```python
from build123d import *

# Parameters (mm, degrees)
BOSS_EXTRUDE1_DEPTH = 19.05
BOSS_EXTRUDE2_DEPTH = 3.175
SKETCH3_R           = 3.175
CUT_EXTRUDE1_DEPTH  = 189.387669682
SKETCH4_W           = 151.529186582
SKETCH4_H           = 154.937341475
CUT_EXTRUDE2_DEPTH  = 146.05


with BuildPart() as part:
    # Sketch1 → Boss-Extrude1 (new body)
    with BuildSketch(Plane.XY):
        Polygon((0, 0), (0, -26.595904174), (100.162396017, -140.692505), (127, -140.692505), (127, -137.517505), (101.6, -137.517505), (3.175, -25.4), (3.175, 0), align=None)
    boss_extrude1 = extrude(amount=BOSS_EXTRUDE1_DEPTH)

    # Sketch2 → Boss-Extrude2 (add)
    with BuildSketch(Plane(origin=(0, 0, 0), x_dir=(-1, 0, 0), z_dir=(0, 0, -1))):
        Polygon((-19.05, 0), (-3.175, 0), (-3.175, -25.4), (-101.6, -137.517505), (-127, -137.517505), (-127, -121.642505), (-108.788019913, -121.642505), (-19.05, -19.42047913), align=None)
    boss_extrude2 = extrude(amount=-BOSS_EXTRUDE2_DEPTH)

    # Sketch3 → Cut-Extrude1 (cut, through all)
    with BuildSketch(Plane(origin=(3.175, 0, 0), x_dir=(0, 0, -1), z_dir=(1, 0, 0))):
        with Locations(Location((-11.1125, -7.690689216, 0), (0, 0, 90))):
            Circle(SKETCH3_R)
    cut_extrude1 = extrude(amount=-CUT_EXTRUDE1_DEPTH, mode=Mode.SUBTRACT)

    # Mirror1: Boss-Extrude1, Boss-Extrude2, Cut-Extrude1 across plane
    add(boss_extrude1.mirror(Plane(origin=(0, 0, 19.05), x_dir=(0, 0, 1), z_dir=(1, 0, 0))))
    add(boss_extrude2.mirror(Plane(origin=(0, 0, 19.05), x_dir=(0, 0, 1), z_dir=(1, 0, 0))))
    add(cut_extrude1.mirror(Plane(origin=(0, 0, 19.05), x_dir=(0, 0, 1), z_dir=(1, 0, 0))), mode=Mode.SUBTRACT)

    # Sketch4 → Cut-Extrude2 (cut)
    with BuildSketch(Plane.XY.offset(19.05)):
        with Locations((75.764593291, -77.468670738)):
            Rectangle(SKETCH4_W, SKETCH4_H)
    extrude(amount=-CUT_EXTRUDE2_DEPTH, mode=Mode.SUBTRACT)


solid = part.part
```
The model under review builds one solid part; all positions refer to its coordinate system, in mm. A direction names the side the tool comes from. Coordinates: 2 decimals unless noted, no trailing zeros. Write each loop counter-clockwise with the first axis right and the second up, starting at its lowest first coordinate (ties: lowest second). Pieces come first, ordered by that corner, then holes. Notation, with made-up numbers: (72, 57.5) - (89, 57.5) arc R16 ccw to (89, 69.5) - close; hole circle Ø1 at (-1, -15). An arc over 180 degrees is marked (long way). Answer in a Markdown table with one row per item. Add a question column.
Q1. Consider section A-A on z = 16.5. Give the boundary of the cut face in (x, y) (1 decimal).
Q2. To check wall thickness, follow line 1 along Z through (x, y) = (-102, -118) (3 decimals); line 2 along X through (y, z) = (-13, 4) (3 decimals); line 3 along Y through (x, z) = (-113, 13.5). State the ranges of each line that lie inside material, in increasing order. Write a range as from..to.
Q3. Draft analysis for pull direction Z (two halves, no side actions). For faces 4 (the face through (-56, -74, 3.175)), 5 (the face through (-7, 0, 2)), 6 (the face through (-1.61, -10.21, 9.18)), state which applies: +Z half, -Z half, draft (parallel to the pull), parting line (faces both ways), or undercut.
Q4. Clearance check with flat-ended pins moving along their axes: pin 1 (3.5 mm diameter, centred on x = -122, z = 1.5, fed in from +Y); pin 2 (2 mm diameter, centred on x = -96, z = 13.5, fed in from -Y); pin 3 (5 mm diameter, centred on x = -109, z = 11, fed in from +Y). State where each tip first meets the part, or that it passes through.
Q5. Consider section D-D on y = -111. Give the boundary of the cut face in (x, z) (3 decimals).
Q6. Consider section B-B on z = 9.5. Give the boundary of the cut face in (x, y) (1 decimal), then the cut area to 3 significant figures.
Q7. For faces 1 (the face through (-114, -137.518, 11)), 2 (the face through (-127, -138, 5)), 3 (the face through (-19.05, -10, 2)), list the 3-axis set-ups (+Z, -Z, +X, -X, +Y, -Y) from which the entire face can be reached by the end or side of a thin tool; tool diameter is ignored.
Answers below:
| question | item | result |
|---|---|---|
| 1 | outline | (-127, -140.7) - (-100.2, -140.7) - (0, -26.6) - (0, 0) - (-3.2, 0) - (-3.2, -25.4) - (-101.6, -137.5) - (-127, -137.5) - close |
| 2 | line 1 | 0..3.175 |
| 2 | line 2 | -3.175..0 |
| 2 | line 3 | -140.69..-137.52 |
| 3 | face 4 | +Z half |
| 3 | face 5 | draft |
| 3 | face 6 | undercut |
| 4 | pin 1 | y = -121.64 |
| 4 | pin 2 | y = -137.09 |
| 4 | pin 3 | y = -137.52 |
| 5 | outline | (-99.445, 0) - (-74.096, 0) - (-74.096, 19.05) - (-78.321, 19.05) - (-78.321, 3.175) - (-99.445, 3.175) - close |
| 6 | outline | (-127, -140.7) - (-100.2, -140.7) - (0, -26.6) - (0, -10.4) - (-3.2, -10.4) - (-3.2, -25.4) - (-101.6, -137.5) - (-127, -137.5) - close; (-3.2, -5) - (0, -5) - (0, 0) - (-3.2, 0) - close |
| 6 | area | 626 mm² |
| 7 | face 1 | +Z, -X, +Y |
| 7 | face 2 | +Z, -Z, -X, +Y, -Y |
| 7 | face 3 | +Z, -Z, -X, +Y |
